```python
from build123d import *

# Parameters (mm, degrees)
SKETCH1_W           = 30
SKETCH1_H           = 25
BOSS_EXTRUDE1_DEPTH = 2
SKETCH2_W           = 5
SKETCH2_H           = 5
BOSS_EXTRUDE2_DEPTH = 1
SKETCH3_R           = 1.5
CUT_EXTRUDE1_DEPTH  = 4


with BuildPart() as part:
    # Sketch1 → Boss-Extrude1 (new body)
    with BuildSketch(Plane(origin=(0, 0, 0), x_dir=(1, 0, 0), z_dir=(0, 1, 0))):
        with Locations((15, 12.5)):
            Rectangle(SKETCH1_W, SKETCH1_H)
    extrude(amount=BOSS_EXTRUDE1_DEPTH)

    # Sketch2 → Boss-Extrude2 (add)
    with BuildSketch(Plane(origin=(0, 2, 0), x_dir=(1, 0, 0), z_dir=(0, 1, 0))):
        with Locations((10.5, 14.5)):
            Rectangle(SKETCH2_W, SKETCH2_H)
    extrude(amount=BOSS_EXTRUDE2_DEPTH)

    # Sketch3 → Cut-Extrude1 (cut)
    with BuildSketch(Plane(origin=(0, 2, 0), x_dir=(1, 0, 0), z_dir=(0, 1, 0))):
        with Locations(Location((3, 22, 0), (0, 0, 270))):
            Circle(SKETCH3_R)
    extrude(amount=-CUT_EXTRUDE1_DEPTH, mode=Mode.SUBTRACT)


solid = part.part
```
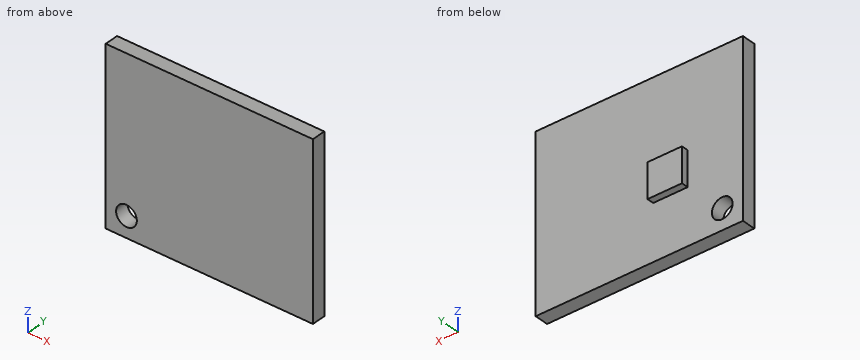
The model under review builds one solid part; all positions refer to its coordinate system, in mm. Round coordinates to 2 decimals unless told otherwise and drop trailing zeros. Order: outer loops, then holes, each group sorted by start corner. A loop starts at its lowest first (then second) coordinate and runs counter-clockwise, first axis right, second up.
Item 1: Add section D-D, the plane x = 21. State the section outline as (y, z) points, and give its area (3 significant figures).
Working result:
outline: (0, -25) - (2, -25) - (2, 0) - (0, 0) - close
area: 50.0 mm2
Item 2: Add section B-B, the plane z = -22. State the section outline as (x, y) points, and give its area (3 significant figures).
Working result:
outline: (0, 0) - (1.5, 0) - (1.5, 2) - (0, 2) - close; (4.5, 0) - (30, 0) - (30, 2) - (4.5, 2) - close
area: 54.0 mm2
Item 3: For pin 1 (0.5 mm diameter, centred on x = 11, y = 2.5, fed in from +Z); pin 2 (0.8 mm diameter, centred on x = 10, y = 2.5, fed in from -Z); pin 3 (0.8 mm diameter, centred on y = 2.5, z = -15, fed in from +X); pin 4 (8 mm diameter, centred on x = 9.5, z = -9.5, fed in from -Y), all flat-tipped, find the tip position at first contact; note any pin that passes through.
Working result:
pin 1: stops at z = -12
pin 2: stops at z = -17
pin 3: stops at x = 13
pin 4: stops at y = 0
Item 4: To check wall thickness, follow probe 1 along X at (y, z) = (1.15, -22); probe 2 along Y at (x, z) = (25, -11). State the ranges of each line that lie inside material, in increasing order.
Working result:
probe 1: x = 0 to 1.5, 4.5 to 30
probe 2: y = 0 to 2
Item 5: Add section C-C, the plane z = -15. State the section outline as (x, y) points.
Working result:
outline: (0, 0) - (30, 0) - (30, 2) - (13, 2) - (13, 3) - (8, 3) - (8, 2) - (0, 2) - close
Item 6: Add section A-A, the plane x = 3. State the section outline as (y, z) points, and give its area (3 significant figures).
Working result:
outline: (0, -25) - (2, -25) - (2, -23.5) - (0, -23.5) - close; (0, -20.5) - (2, -20.5) - (2, 0) - (0, 0) - close
area: 44.0 mm2
